```python
from build123d import *

# Parameters (mm, degrees)
F0_W     = 914.4
F0_H     = 876.3
F1_DEPTH = 30.226
F2_W     = 28.575
F2_H     = 876.3
F3_DEPTH = 2292.35
F5_DEPTH = 876.3


with BuildPart() as f1:
    # F0 (on Right) → F1 (new body)
    with BuildSketch(Plane.YZ):
        Rectangle(F0_W, F0_H)
    extrude(amount=F1_DEPTH)

    # F2 (on face) → F3 (join)
    with BuildSketch(Plane.YZ.offset(30.226)):
        with Locations((-239.7125, 0)):
            Rectangle(F2_W, F2_H)
    extrude(amount=F3_DEPTH)

    # F4 (on face) → F5 (join)
    with BuildSketch(Plane.XY.offset(438.15)):
        Polygon((2322.576, -225.425), (2322.576, -254), (2322.576, -457.2), (2352.802, -457.2), (2352.802, 457.2), (2322.576, 457.2), align=None)
    extrude(amount=-F5_DEPTH)


solid = f1.part
```
Input: part model. Units: mm. Frame: model coordinates. A direction names the side the tool comes from. Coordinates: 2 decimals unless noted, no trailing zeros. Write each loop counter-clockwise with the first axis right and the second up, starting at its lowest first coordinate (ties: lowest second). Pieces come first, ordered by that corner, then holes.
1) Section B-B on z = -142. Output: boundary loops of the cut face in (x, y) (3 decimals).
2) Section A-A on y = 48. Output: boundary loops of the cut face in (x, z), and give its area (3 significant figures).
3) Mould query, pull axis X, two halves, no side actions, for faces 4 (the flat face through (2352.802, -6, 6)), 5 (the flat face through (1160, -254, -6)), 6 (the flat face through (1171, -235, 438.15)). Classes: pulls with the +X half, pulls with the -X half, needs draft (parallel to the pull), parting line crosses it, or undercut.
4) Set-up query: faces 1 (the flat face through (0, -6, 6)), 2 (the flat face through (2322.576, -354, 6)), 3 (the flat face through (2322.576, 121, 6)). Return all of +Z, -Z, +X, -X, +Y, -Y with unobstructed straight access to the full face (end or side cutting, diameter ignored); none if empty.
5) Material intervals for line 1 along X through (y, z) = (-132, -211); line 2 along Y through (x, z) = (1415.5, 397) (3 decimals), sorted ascending.
6) Section C-C on x = 379. Output: boundary loops of the cut face in (y, z) (3 decimals), and give its area (3 significant figures).
7) Pin query (flat end, axial travel): pin 1 Ø6 at (x, z) = (641, -130.5) entering from -Y. Return the tip coordinate at first contact, or that it passes through.
Check result:
1. outline: (0, -457.2) - (30.226, -457.2) - (30.226, -254) - (2322.576, -254) - (2322.576, -457.2) - (2352.802, -457.2) - (2352.802, 457.2) - (2322.576, 457.2) - (2322.576, -225.425) - (30.226, -225.425) - (30.226, 457.2) - (0, 457.2) - close
2. outline: (0, -438.15) - (30.23, -438.15) - (30.23, 438.15) - (0, 438.15) - close; (2322.58, -438.15) - (2352.8, -438.15) - (2352.8, 438.15) - (2322.58, 438.15) - close
2. area: 53,000 mm2
3. face 4: pulls with the +X half
3. face 5: undercut
3. face 6: needs draft
4. face 1: +Z, -Z, -X, +Y, -Y
4. face 2: +Z, -Z, -Y
4. face 3: +Z, -Z, +Y
5. line 1: x = 0 to 30.23, 2322.58 to 2352.8
5. line 2: y = -254 to -225.425
6. outline: (-254, -438.15) - (-225.425, -438.15) - (-225.425, 438.15) - (-254, 438.15) - close
6. area: 25,000 mm2
7. pin 1: stops at y = -254
